from build123d import *

# Parameters (mm, degrees)
EXTRUDE_1_DEPTH          = 2.45
CUT_EXTRUDE_1_DEPTH      = 3.1
CUT_EXTRUDE_1_DEPTH_BACK = 3.1
SKETCH_4_R               = 1
CUT_EXTRUDE_2_DEPTH      = 6.1
CHAMFER_1_SIZE           = 1


with BuildPart() as part:
    # 草图1 → 凸台-拉伸1 (new body)
    with BuildSketch(Plane.XY):
        with BuildLine():
            Line((-6.9, 6.9), (6.9, 6.9))
            ThreePointArc((6.9, 6.9), (7.607106781, 6.607106781), (7.9, 5.9))
            Line((7.9, 5.9), (7.9, -5.9))
            ThreePointArc((7.9, -5.9), (7.607106781, -6.607106781), (6.9, -6.9))
            Line((6.9, -6.9), (-6.9, -6.9))
            ThreePointArc((-6.9, -6.9), (-7.607106781, -6.607106781), (-7.9, -5.9))
            Line((-7.9, -5.9), (-7.9, 5.9))
            ThreePointArc((-7.9, 5.9), (-7.607106781, 6.607106781), (-6.9, 6.9))
        make_face()
    extrude(amount=EXTRUDE_1_DEPTH)

    # 草图3 → 切除-拉伸1 (cut, two sides: drawn at the far end of the back side and taken through both)
    with BuildSketch(Plane(origin=(0, 0, 0), x_dir=(0, 0, -1), z_dir=(1, 0, 0)).offset(-CUT_EXTRUDE_1_DEPTH_BACK)):
        with BuildLine():
            Line((0.008677119, -0.72827251), (0.008677119, 0.77172749))
            ThreePointArc((0.008677119, 0.77172749), (-0.741322881, 0.02172749), (0.008677119, -0.72827251))
        make_face()
        with BuildLine():
            Line((0.008677119, -6.72827251), (0.008677119, -5.22827251))
            ThreePointArc((0.008677119, -5.22827251), (-0.741322881, -5.97827251), (0.008677119, -6.72827251))
        make_face()
        with BuildLine():
            Line((0.008677119, -4.72827251), (0.008677119, -3.22827251))
            ThreePointArc((0.008677119, -3.22827251), (-0.741322881, -3.97827251), (0.008677119, -4.72827251))
        make_face()
        with BuildLine():
            Line((0.008677119, -2.72827251), (0.008677119, -1.22827251))
            ThreePointArc((0.008677119, -1.22827251), (-0.741322881, -1.97827251), (0.008677119, -2.72827251))
        make_face()
        with BuildLine():
            Line((0.008677119, 1.27172749), (0.008677119, 2.77172749))
            ThreePointArc((0.008677119, 2.77172749), (-0.741322881, 2.02172749), (0.008677119, 1.27172749))
        make_face()
        with BuildLine():
            Line((0.008677119, 3.27172749), (0.008677119, 4.77172749))
            ThreePointArc((0.008677119, 4.77172749), (-0.741322881, 4.02172749), (0.008677119, 3.27172749))
        make_face()
        with BuildLine():
            Line((0.008677119, 5.27172749), (0.008677119, 6.77172749))
            ThreePointArc((0.008677119, 6.77172749), (-0.741322881, 6.02172749), (0.008677119, 5.27172749))
        make_face()
    extrude(amount=CUT_EXTRUDE_1_DEPTH + CUT_EXTRUDE_1_DEPTH_BACK, mode=Mode.SUBTRACT)

    # 草图4 → 切除-拉伸2 (cut)
    with BuildSketch(Plane.XY.offset(2.45)):
        with Locations((-5, -4)):
            Circle(SKETCH_4_R)
        with Locations((4.96323916, -4)):
            Circle(SKETCH_4_R)
        with Locations((4.96323916, 4.01838042)):
            Circle(SKETCH_4_R)
        with Locations((-5, 4.01838042)):
            Circle(SKETCH_4_R)
    extrude(amount=-CUT_EXTRUDE_2_DEPTH, mode=Mode.SUBTRACT)

    # 倒角1
    chamfer_1_edges = [part.edges().sort_by_distance(p)[0] for p in [
        (-6, 4.01838042, 2.45),
        (3.96323916, 4.01838042, 2.45),
        (3.96323916, -4, 2.45),
        (-6, -4, 2.45),
    ]]
    chamfer(chamfer_1_edges, length=CHAMFER_1_SIZE)


solid = part.part
Verification items for the finished model (mm, model axes). A direction names the side the tool comes from. Coordinates: 2 decimals unless noted, no trailing zeros. Order: outer loops, then holes, each group sorted by start corner. A loop starts at its lowest first (then second) coordinate and runs counter-clockwise, first axis right, second up. Notation, with made-up numbers: (-12.5, 5.5) -> (-8.5, 5.5) arc R5 ccw to (-8.5, 10.5) -> close; hole circle Ø4 at (51.5, 32). An arc over 180 degrees is marked (long way). Put each result on its own line as item: value. Start each with the question number.
1. Material ranges on L1, parallel to Y at x = -5.5, z = 1.35; L2, parallel to X at y = 4.75, z = 0.85; L3, parallel to Y at x = -6.5, z = 2.1, recorded low to high. Write a range as [from, to].
2. Mould release check, pull along Y, two halves, no side actions. Record for faces 3 (the cylindrical face through (4.226, 4.694, 0.735)), 4 (the flat face through (0, 6.9, 1)), 5 (the flat face through (-7.9, 0, 1)): released by +Y, released by -Y, zero draft, split by the parting line, or undercut.
3. Go/stop test with flat-tipped pins: pin 1 Ø2.5 at (x, y) = (-5, -4) entering from +Z; pin 2 Ø0.6 at (y, z) = (-6.5, 0.5) entering from +X; pin 3 Ø2 at (x, y) = (5.5, 4.5) entering from +Z. Record where each tip stops, or that it passes through.
4. Cross-section at B-B, the plane x = 0.75. Record the boundary of the cut face in (y, z), then the cut area to 3 significant figures.
5. Cross-section at C-C, the plane y = -4. Record the boundary of the cut face in (x, z).
6. Access from +Z, -Z, +X, -X, +Y, -Y to the whole of each face (thin tool, end or side, straight path). Record for faces 1 (the cylindrical face through (-5.13, 5.01, 0.74)), 2 (the cylindrical face through (-0.04, -3.96, 0.74)).
7. Cross-section at D-D, the plane z = 0.5. Count the separate pieces of the cut face and the enclosed holes in it, then the cut area to 3 significant figures.
8. Cross-section at A-A, the plane x = -5. Record the boundary of the cut face in (y, z), then the cut area to 3 significant figures.
Computed:
1. L1: [-6.9, -4.87], [-3.13, 3.15], [4.88, 6.9]
1. L2: [-7.9, -5.68], [-4.32, 4.28], [5.64, 7.9]
1. L3: [-6.9, -4.69], [-3.31, 3.33], [4.71, 6.9]
2. face 3: undercut
2. face 4: released by +Y
2. face 5: zero draft
3. pin 1: z = 1.7
3. pin 2: x = 7.85
3. pin 3: z = 2.17
4. outline: (-6.9, 0) -> (-6.73, 0) arc R0.75 cw to (-5.23, 0) -> (-4.73, 0) arc R0.75 cw to (-3.23, 0) -> (-2.73, 0) arc R0.75 cw to (-1.23, 0) -> (-0.73, 0) arc R0.75 cw to (0.77, 0) -> (1.27, 0) arc R0.75 cw to (2.77, 0) -> (3.27, 0) arc R0.75 cw to (4.77, 0) -> (5.27, 0) arc R0.75 cw to (6.77, 0) -> (6.9, 0) -> (6.9, 2.45) -> (-6.9, 2.45) -> close
4. area: 27.7 mm2
5. outline: (-7.9, 0) -> (-6, 0) -> (-6, 1.45) -> (-7, 2.45) -> (-7.9, 2.45) -> close; (-4, 0) -> (-3.1, 0) -> (-3.1, 0.74) -> (3.1, 0.74) -> (3.1, 0) -> (3.96, 0) -> (3.96, 1.45) -> (2.96, 2.45) -> (-3, 2.45) -> (-4, 1.45) -> close; (5.96, 0) -> (7.9, 0) -> (7.9, 2.45) -> (6.96, 2.45) -> (5.96, 1.45) -> close
6. face 1: +Z, -Z
6. face 2: -Z
7. separate pieces: 1
7. enclosed holes: 11
7. area: 157 mm2
8. outline: (-6.9, 0) -> (-5, 0) -> (-5, 1.45) -> (-6, 2.45) -> (-6.9, 2.45) -> close; (-3, 0) -> (3.02, 0) -> (3.02, 1.45) -> (2.02, 2.45) -> (-2, 2.45) -> (-3, 1.45) -> close; (5.02, 0) -> (6.9, 0) -> (6.9, 2.45) -> (6.02, 2.45) -> (5.02, 1.45) -> close
8. area: 22.0 mm2
